Geometry check sheet. Reference: the model listing, model coordinates, mm. A direction names the side the tool comes from. Round coordinates to 2 decimals unless told otherwise and drop trailing zeros. Write each loop counter-clockwise with the first axis right and the second up, starting at its lowest first coordinate (ties: lowest second). Pieces come first, ordered by that corner, then holes. Notation, with made-up numbers: M 34,1 L 54,1 A19 ccw 54,6 Z; hole C 34,60.25 d10. An arc over 180 degrees is marked long. Put each result on its own line as item: value. Start each with the question number.
(1) Tool access check on faces 1 (the flat face through (5, -24, 87)), 2 (the flat face through (24, 5, 87)), 3 (the flat face through (0, 0, 0)), 4 (the cylindrical face through (18.475, -7.66, 77.638)). Record the directions out of +Z, -Z, +X, -X, +Y, -Y that give a thin tool (end or side, any length) a straight path to the whole face; none if there is none.
(2) Mould release check, pull along X, two halves, no side actions. Record for faces 5 (the flat face through (10, 23, 90)), 6 (the flat face through (20.79, 13.72, 87.46)), 7 (the flat face through (20.79, -13.72, 87.46)): pulls with the +X half, pulls with the -X half, needs draft (parallel to the pull), parting line crosses it, or undercut.
(3) Section check B-B on x = -4. Record the cut outline in (y, z).
(4) Section check C-C on z = 71. Record the cut outline in (x, y).
(5) Section check A-A on y = 0. Record the cut outline in (x, z).
(6) Section check D-D on z = 54. Record the cut outline in (x, y).
(7) Gauge pin test, flat ends, axial feed: pin 1 (2.5 mm diameter, centred on y = 26.5, z = 86.5, fed in from +X); pin 2 (11 mm diameter, centred on x = 0.5, y = -26, fed in from +Z); pin 3 (3 mm diameter, centred on x = -22.5, y = 2, fed in from +Z); pin 4 (6 mm diameter, centred on y = -12, z = 26.5, fed in from +X). Record the tip position at first contact, or that the pin passes through.
(8) Material ranges on probe 1 along Y at (x, z) = (0, 83.25); probe 2 along Z at (x, y) = (-19, 18); probe 3 along Z at (x, y) = (3.5, 19), recorded low to high.
from build123d import *

# Parameters (mm, degrees)
BOX_W             = 15
BOX_H             = 10
BOX_DEPTH         = 10
ARRAY_COUNT       = 8
CYLINDER001_R     = 20
CYLINDER001_DEPTH = 20
CYLINDER_R        = 30
CYLINDER_DEPTH    = 90


with BuildPart() as array:
    # Box → Box (new body)
    with BuildSketch(Plane(origin=(19, -5, 85), x_dir=(1, 0, 0), z_dir=(0, 0, 1))):
        with Locations((7.5, 5)):
            Rectangle(BOX_W, BOX_H)
    extrude(amount=BOX_DEPTH)

    # Array: Array ×8 about axis
    array_axis = Axis((0, 0, 0), (0, 0, 1))


with BuildPart() as array_1:
    add(array.part)
    for i in range(1, ARRAY_COUNT):
        add(array.part.rotate(array_axis, i * 360 / ARRAY_COUNT))


with BuildPart() as obj1:
    # Cylinder001 → Cylinder001 (new body)
    with BuildSketch(Plane.XY.offset(70)):
        Circle(CYLINDER001_R)
    extrude(amount=CYLINDER001_DEPTH)


with BuildPart() as cut001:
    # Cylinder → Cylinder (new body)
    with BuildSketch(Plane.XY):
        Circle(CYLINDER_R)
    extrude(amount=CYLINDER_DEPTH)

    # Cut: cut obj1
    add(obj1.part, mode=Mode.SUBTRACT)

    # Cut001: cut Array
    add(array_1.part, mode=Mode.SUBTRACT)


solid = cut001.part
Answers follow:
1. face 1: +Z, +Y, -Y
1. face 2: +Z, +X, -X
1. face 3: -Z, +X, -X, +Y, -Y
1. face 4: +Z
2. face 5: needs draft
2. face 6: undercut
2. face 7: undercut
3. outline: M -29.73,0 L 29.73,0 L 29.73,85 L 19.6,85 L 19.6,70 L -19.6,70 L -19.6,85 L -29.73,85 Z
4. outline: C 0,0 d60; hole C 0,0 d40
5. outline: M -30,0 L 30,0 L 30,85 L 20,85 L 20,70 L -20,70 L -20,85 L -30,85 Z
6. outline: C 0,0 d60
7. pin 1: stops at x = 16.2
7. pin 2: stops at z = 90
7. pin 3: stops at z = 85
7. pin 4: stops at x = 28.62
8. probe 1: y = -30 to -20, 20 to 30
8. probe 2: z = 0 to 85
8. probe 3: z = 0 to 70
